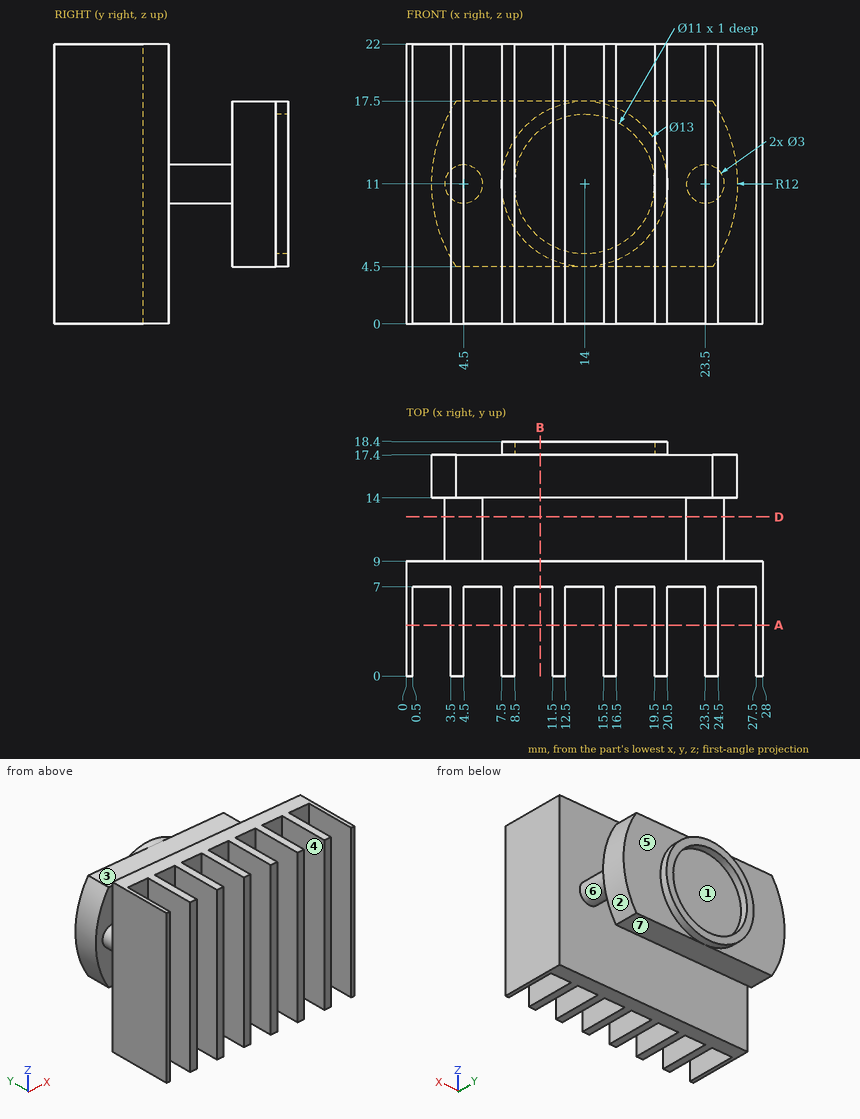
Could you check a few things on this drawing? It's one solid part, dimensions in mm from its lowest x, y, z. A direction names the side the tool comes from. Give positions to 0.01 mm unless a question says otherwise; leave off trailing zeros. Order: outer loops, then holes, each group sorted by start corner. A loop starts at its lowest first (then second) coordinate and runs counter-clockwise, first axis right, second up. Notation, with made-up numbers: (64.5, 39.5) -> (114.5, 39.5) arc R12 cw to (114.5, 54.5) -> close; hole circle Ø8 at (-2, 34). An arc over 180 degrees is marked (long way). Use CSV: the item, a comma, the result in double quotes. Start each with the question number.
Item 1: I'm going to push flat-ended pins straight in: P1, Ø4, axis at y = 14, z = 18.5, coming from the +X side; P2, Ø2.5, axis at x = 14, y = 16.5, coming from the -Z side; P3, Ø1.5, axis at x = 10.5, z = 13.5, coming from the -Y side. Where does each tip first touch, or does it pass through?
Item 2: Suppose I cut it at B-B (x = 10.5). List the corners of the cut face in (y, z) for me.
Item 3: On a 3-axis mill with a long thin cutter (end or side, diameter ignored), from which of +Z, -Z, +X, -X, +Y, -Y can I reach the whole of each face in a straight line? I mean the marked faces 1, 2, 3 and 4. Say none if no direction works.
Item 4: Suppose I cut it at D-D (y = 12.5). List the corners of the cut face in (x, z) for me, and give its area (3 significant figures).
Item 5: If I drill on probe 1 along X at (y, z) = (18, 11); probe 2 along Y at (x, z) = (21.25, 5.75); probe 3 along X at (y, z) = (11.5, 11), over which ranges is the centre line in solid material (lowest first)? Write a range as [from, to].
Item 6: Suppose I cut it at A-A (y = 4). Give the number of separate pieces and of enclosed holes in the cut face, and give its area (3 significant figures).
Item 7: Thinking about a two-plate mould opening in Y: for the marked faces 5, 6 and 7, which applies, pulls with the +Y half, pulls with the -Y half, needs draft (parallel to the pull), parting line crosses it, or undercut?
Answer block:
1,P1,"stops at x = 24.67"
1,P2,"stops at z = 4.5"
1,P3,"stops at y = 7"
2,outline,"(7, 0) -> (9, 0) -> (9, 22) -> (7, 22) -> close; (14, 4.5) -> (17.4, 4.5) -> (17.4, 5.52) -> (18.4, 5.52) -> (18.4, 6.76) -> (17.4, 6.76) -> (17.4, 15.24) -> (18.4, 15.24) -> (18.4, 16.48) -> (17.4, 16.48) -> (17.4, 17.5) -> (14, 17.5) -> close"
3,face 1,"+Y"
3,face 2,"+X, +Y"
3,face 3,"+Z, +X, -X, +Y"
3,face 4,"+Z, -Z, -Y"
4,outline,"circle Ø3 at (4.5, 11); circle Ø3 at (23.5, 11)"
4,area,"14.1 mm^2"
5,probe 1,"x = [7.5, 8.5], [19.5, 20.5]"
5,probe 2,"y = [7, 9], [14, 17.4]"
5,probe 3,"x = [3, 6], [22, 25]"
6,separate pieces,"8"
6,enclosed holes,"0"
6,area,"154 mm^2"
7,face 5,"pulls with the +Y half"
7,face 6,"undercut"
7,face 7,"needs draft"
